Geometry check sheet. Reference: the model listing, model coordinates, mm. Face numbers are marked on the shaded views. A direction names the side the tool comes from. Coordinates: 2 decimals unless noted, no trailing zeros. Loops run counter-clockwise (first coordinate to the right, second up) from the corner with the lowest first, then second, coordinate; pieces in that order, holes last. Notation, with made-up numbers: (48, 44.25) - (76, 44.25) arc R22 ccw to (76, 70.25) - close; hole circle Ø10 at (64.25, 54.25). An arc over 180 degrees is marked (long way). Write each question's results on one line, items separated by ' | '. Start each with the question number.
(1) Access from +Z, -Z, +X, -X, +Y, -Y to the whole of each face (thin tool, end or side, straight path). Record for the marked faces 1 and 2.
(2) Go/stop test with flat-tipped pins: pin 1 Ø6 at (y, z) = (16, 3.5) entering from +X; pin 2 Ø10 at (x, z) = (0.5, 4) entering from -Y; pin 3 Ø6 at (x, y) = (9, 24) entering from +Z. Record where each tip stops, or that it passes through.
(3) Sectioned sample at B-B (x = 8). Enter the section's corners in (y, z).
(4) Sectioned sample at A-A (y = 5). Enter the section's corners in (x, z).
(5) Material ranges on probe 1 along Z at (x, y) = (4.5, 13.5); probe 2 along X at (y, z) = (26.5, 2.5), recorded low to high.
(6) Sectioned sample at C-C (z = 6). Enter the section's corners in (x, y).
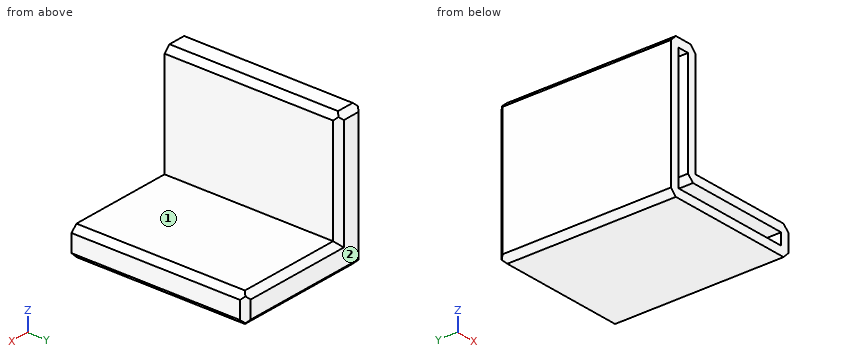
Solid Edge part; units mm, degrees
sketch "Sketch1" plane through (0, 0, 0) normal (0, -1, 0) x (1, 0, 0)
  line L0 (12, 12) -> (-12, 12)
  line L1 (-12, 12) -> (-12, -12)
  line L2 (-12, -12) -> (12, -12)
  line L3 (12, -12) -> (12, 12)
extrude "Protrusion1" add sketch "Sketch1" against normal blind 30
sketch "Sketch2" plane through (0, 0, 0) normal (0, -1, 0) x (1, 0, 0)
  line L0 (-8.5, 10.5) -> (-8.5, -8.5)
  line L1 (-8.5, -8.5) -> (10.5, -8.5)
  line L2 (10.5, -8.5) -> (10.5, -10.5)
  line L3 (10.5, -10.5) -> (-10.5, -10.5)
  line L4 (-10.5, -10.5) -> (-10.5, 10.5)
  line L5 (-10.5, 10.5) -> (-8.5, 10.5)
extrude "VaciadoExtruido_1" cut sketch "Sketch2" against normal blind 25
sketch "Sketch3" plane through (0, 0, 0) normal (0, -1, 0) x (1, 0, 0)
  line L0 (-7, 12) -> (-7, -7)
  line L1 (-7, -7) -> (12, -7)
extrude "Cutout1" cut sketch "Sketch3" against normal through all material side at (-6.95, 0, 2.5)
chamfer "Chaflán_1" distance 1 angle 45 6 edges at (-12, 15, 12) (-7, 15, 12) (-12, 15, -12) (12, 15, -12) (12, 15, -7) (-8.5, 12.5, -8.5)
chamfer "Chaflán_2" distance 1 angle 45 6 edges at (-9.5, 30, 12) (-12, 30, 0) (-7, 30, 2) (2, 30, -7) (12, 30, -9.5) (0, 30, -12)
Outcome:
1) face 1: +Z, +X, +Y, -Y | face 2: +Z, -Z, +X, -X, +Y
2) pin 1: stops at x = -7 | pin 2: passes through | pin 3: stops at z = -7
3) outline: (0, -12) - (29, -12) - (30, -11) - (30, -8) - (29, -7) - (0, -7) - (0, -8.5) - (25, -8.5) - (25, -10.5) - (0, -10.5) - close
4) outline: (-12, -11) - (-11, -12) - (11, -12) - (12, -11) - (12, -8) - (11, -7) - (-7, -7) - (-7, 11) - (-8, 12) - (-11, 12) - (-12, 11) - close; hole (-10.5, -10.5) - (10.5, -10.5) - (10.5, -8.5) - (-7.5, -8.5) - (-8.5, -7.5) - (-8.5, 10.5) - (-10.5, 10.5) - close
5) probe 1: z = -12 to -10.5, -8.5 to -7 | probe 2: x = -12 to -7
6) outline: (-12, 0) - (-10.5, 0) - (-10.5, 25) - (-8.5, 25) - (-8.5, 0) - (-7, 0) - (-7, 29) - (-8, 30) - (-11, 30) - (-12, 29) - close
